Autodesk Inventor part; units mm, degrees
ref_plane "YZ Plane" through (0, 0, 0) normal (1, 0, 0) x (0, 1, 0)
ref_plane "XZ Plane" through (0, 0, 0) normal (0, 1, 0) x (-1, 0, 0)
ref_plane "XY Plane" through (0, 0, 0) normal (0, 0, 1) x (1, 0, 0)
sketch "Sketch1" plane through (0, 0, 0) normal (0, 1, 0) x (-1, 0, 0)
  line L0 (-50, -50) -> (50, -50)
  line L1 (50, -50) -> (50, 50)
  line L2 (50, 50) -> (-50, 50)
  line L3 (-50, 50) -> (-50, -50)
  line L4 (-50, -50) -> (50, 50) construction
  line L5 (50, -50) -> (-50, 50) construction
  point P0 (0, 0)
  dimension "d0" = 100
  dimension "d1" = 100
extrude "Extrusion1" add sketch "Sketch1" along normal blind 5
sketch "Sketch2" plane through (0, 0, 0) normal (0, -1, 0) x (1, 0, 0)
  line L0 (50, 50) -> (50, -50)
  line L1 (-50, -4) -> (50, -4)
  line L2 (50, -4) -> (50, 4)
  line L3 (50, 4) -> (-50, 4)
  line L4 (-50, 4) -> (-50, -4)
  line L5 (-50, -4) -> (50, 4) construction
  line L6 (50, -4) -> (-50, 4) construction
  point P0 (0, 0)
  dimension "d4" = 8
extrude "Extrusion2" add sketch "Sketch2" along normal blind 4
sketch "Sketch3" plane through (0, 5, 0) normal (0, 1, 0) x (1, 0, 0)
  point P0 (0, 0)
  point P1 (0, 0)
hole "Hole1" at (0, 5, 0) direction (0, -1, 0) diameter 8.5 depth 9
fillet "Fillet1" radius 5 4 edges at (50, 2.5, 50) (50, 2.5, -50) (-50, 2.5, 50) (-50, 2.5, -50)
sketch "Sketch7" plane through (0, 5, 0) normal (0, 1, 0) x (1, 0, 0)
  line L0 (40, -40) -> (-40, -40) construction
  line L1 (-40, -40) -> (-40, 40) construction
  line L2 (-40, 40) -> (40, 40) construction
  line L3 (40, 40) -> (40, -40) construction
  circle A0 centre (0, 0) radius 4.25 construction
  line L4 (40, -40) -> (-40, 40) construction
  line L5 (-40, -40) -> (40, 40) construction
  dimension "d27" = 80
  dimension "d28" = 80
hole "Hole2" at (-40, 5, 40) at (40, 5, -40) at (40, 5, 40) at (-40, 5, -40) direction (0, -1, 0) diameter 10 depth 3
fillet "Fillet2" radius 4 2 edges at (50, -4, 0) (-50, -4, 0)
sketch "Sketch9" plane through (0, 5, 0) normal (0, 1, 0) x (1, 0, 0)
  line L0 (10, 10) -> (-10, 10)
  line L1 (-10, 10) -> (-10, -10)
  line L2 (-10, -10) -> (10, -10)
  line L3 (10, -10) -> (10, 10)
  line L4 (10, 10) -> (-10, -10) construction
  line L5 (-10, 10) -> (10, -10) construction
  point P0 (0, 0)
  dimension "d38" = 20
  dimension "d39" = 20
extrude "Extrusion6" cut sketch "Sketch9" against normal blind 1
properties part number "sliding_platform_3DPrint"
Design review of the part built by this model. Coordinates are the model's own, in mm. A direction names the side the tool comes from. Coordinates: 2 decimals unless noted, no trailing zeros. Loops run counter-clockwise (first coordinate to the right, second up) from the corner with the lowest first, then second, coordinate; pieces in that order, holes last. Notation, with made-up numbers: M 42,1 L 64,1 A6 cw 64,8 Z; hole C 71.5,76 d2. An arc over 180 degrees is marked long. Use one line per item in the form item = value.
(1) For line 1 along X through (y, z) = (3.2, 40); line 2 along Z through (x, y) = (0, 1.5), list the stretches that pass through material, from the lowest coordinate up. Write a range as from..to.
Return value:
line_1 = -50..-45, -35..35, 45..50
line_2 = -50..-4.25, 4.25..50
(2) For faces 4 (the face through (1, 0, 27)), 5 (the face through (-40, 2, -40)), 6 (the face through (1, 0, -27)), list the 3-axis set-ups (+Z, -Z, +X, -X, +Y, -Y) from which the entire face can be reached by the end or side of a thin tool; tool diameter is ignored.
Return value:
face_4 = +Z, +X, -X, -Y
face_5 = +Y
face_6 = -Z, +X, -X, -Y
(3) Consider section B-B (y = -2). Write out the cut boundary in (x, z).
Return value:
outline = M -49.46,-4 L -1.44,-4 A4.25 cw -1.44,4 L -49.46,4 Z; M 1.44,-4 L 49.46,-4 L 49.46,4 L 1.44,4 A4.25 cw Z
(4) Consider section D-D (x = -17). Write out the cut boundary in (y, z), and give its area (3 significant figures).
Return value:
outline = M -4,-4 L 0,-4 L 0,-50 L 5,-50 L 5,50 L 0,50 L 0,4 L -4,4 Z
area = 532 mm2
(5) Draft analysis for pull direction Z (two halves, no side actions). For faces 1 (the face through (49, 3, -48)), 2 (the face through (-48.797, -2.859, -0.056)), 3 (the face through (40, 2, 40)), state which applies: pulls with the +Z half, pulls with the -Z half, needs draft (parallel to the pull), parting line crosses it, or undercut.
Return value:
face_1 = pulls with the -Z half
face_2 = needs draft
face_3 = undercut
(6) Consider section C-C (z = 40). Write out the cut boundary in (x, y).
Return value:
outline = M -50,0 L 50,0 L 50,5 L 45,5 L 45,2 L 35,2 L 35,5 L -35,5 L -35,2 L -45,2 L -45,5 L -50,5 Z
(7) Consider section A-A (x = 0). Write out the cut boundary in (y, z).
Return value:
outline = M 0,-50 L 5,-50 L 5,-10 L 4,-10 L 4,-4.25 L 0,-4.25 Z; M 0,4.25 L 4,4.25 L 4,10 L 5,10 L 5,50 L 0,50 Z
(8) Clearance check with flat-ended pins moving along their axes: P1, Ø8, axis at x = -39.5, z = -42, coming from the +Y side; P2, Ø4.5, axis at x = -19, y = -2.5, coming from the +Z side; P3, Ø1, axis at x = -18.5, z = 39, coming from the -Y side; P4, Ø8, axis at x = -40, z = -40, coming from the +Y side. State where each tip first meets the part, or that it passes through.
Return value:
P1 = 5
P2 = 4
P3 = 0
P4 = 2
